from build123d import *

# Parameters (mm, degrees)
CUT_EXTRUDE1_REACH  = 155.838
SKETCH2_R           = 1.5
SKETCH3_R           = 110
SKETCH3_R_2         = 85
SKETCH3_R_3         = 2.5
BOSS_EXTRUDE1_DEPTH = 5


with BuildPart() as part:
    # Sketch1 → Revolve1 (revolve)
    with BuildSketch(Plane.XY, mode=Mode.PRIVATE) as revolve1_sk:
        Polygon((80, 0), (80, 88), (6, 88), (6, 96), (25, 96), (25, 93), (35, 93), (35, 100), (85, 100), (85, 0), align=None)
    revolve(revolve1_sk.sketch.rotate(Axis((0, 0, 0), (0, 1, 0)), 90), axis=Axis((0, 0, 0), (0, 1, 0)))

    # Sketch2 → Cut-Extrude1 (cut, up to next)
    with BuildSketch(Plane(origin=(0, 96, 0), x_dir=(1, 0, 0), z_dir=(0, 1, 0)), mode=Mode.PRIVATE) as cut_extrude1_sk1:
        with Locations(Location((0, 10.052527236, 0), (0, 0, 270))):
            Circle(SKETCH2_R)
    cut_extrude1_tool1 = extrude(cut_extrude1_sk1.sketch, amount=-CUT_EXTRUDE1_REACH, mode=Mode.PRIVATE) & part.part
    # Sketch2 → Cut-Extrude1 (cut, up to next)
    with BuildSketch(Plane(origin=(0, 96, 0), x_dir=(1, 0, 0), z_dir=(0, 1, 0)), mode=Mode.PRIVATE) as cut_extrude1_sk2:
        with Locations(Location((-9.888059839, -1.883815278, 0), (0, 0, 270))):
            Circle(SKETCH2_R)
    cut_extrude1_tool2 = extrude(cut_extrude1_sk2.sketch, amount=-CUT_EXTRUDE1_REACH, mode=Mode.PRIVATE) & part.part
    # Sketch2 → Cut-Extrude1 (cut, up to next)
    with BuildSketch(Plane(origin=(0, 96, 0), x_dir=(1, 0, 0), z_dir=(0, 1, 0)), mode=Mode.PRIVATE) as cut_extrude1_sk3:
        with Locations(Location((-4.4752587, -16.407987676, 0), (0, 0, 270))):
            Circle(SKETCH2_R)
    cut_extrude1_tool3 = extrude(cut_extrude1_sk3.sketch, amount=-CUT_EXTRUDE1_REACH, mode=Mode.PRIVATE) & part.part
    # Sketch2 → Cut-Extrude1 (cut, up to next)
    with BuildSketch(Plane(origin=(0, 96, 0), x_dir=(1, 0, 0), z_dir=(0, 1, 0)), mode=Mode.PRIVATE) as cut_extrude1_sk4:
        with Locations(Location((15.268544691, 7.491431306, 0), (0, 0, 270))):
            Circle(SKETCH2_R)
    cut_extrude1_tool4 = extrude(cut_extrude1_sk4.sketch, amount=-CUT_EXTRUDE1_REACH, mode=Mode.PRIVATE) & part.part
    add(cut_extrude1_tool1.solids().sort_by_distance((0, 96, -10.052527))[0], mode=Mode.SUBTRACT)
    add(cut_extrude1_tool2.solids().sort_by_distance((-9.88806, 96, 1.883815))[0], mode=Mode.SUBTRACT)
    add(cut_extrude1_tool3.solids().sort_by_distance((-4.475259, 96, 16.407988))[0], mode=Mode.SUBTRACT)
    add(cut_extrude1_tool4.solids().sort_by_distance((15.268545, 96, -7.491431))[0], mode=Mode.SUBTRACT)

    # Sketch3 → Boss-Extrude1 (add)
    with BuildSketch(Plane.XZ):
        with Locations(Location((0, 0, 0), (0, 0, 270))):
            Circle(SKETCH3_R)
        with Locations(Location((0, 0, 0), (0, 0, 270))):
            Circle(SKETCH3_R_2, mode=Mode.SUBTRACT)
        with Locations(Location((0, 97.5, 0), (0, 0, 270))):
            Circle(SKETCH3_R_3, mode=Mode.SUBTRACT)
        with Locations(Location((97.5, 0, 0), (0, 0, 270))):
            Circle(SKETCH3_R_3, mode=Mode.SUBTRACT)
        with Locations(Location((0, -97.5, 0), (0, 0, 270))):
            Circle(SKETCH3_R_3, mode=Mode.SUBTRACT)
        with Locations(Location((-97.5, 0, 0), (0, 0, 270))):
            Circle(SKETCH3_R_3, mode=Mode.SUBTRACT)
    extrude(amount=-BOSS_EXTRUDE1_DEPTH)


solid = part.part
Source: CAD feature listing. Evaluate the final solid. Frame: model axes, mm. A direction names the side the tool comes from. Coordinates: 2 decimals unless noted, no trailing zeros. Loops run counter-clockwise (first coordinate to the right, second up) from the corner with the lowest first, then second, coordinate; pieces in that order, holes last. Notation, with made-up numbers: (62.5, -8) -> (94.5, -8) arc R24 ccw to (94.5, 8) -> close; hole circle Ø6 at (54.25, 50). An arc over 180 degrees is marked (long way). Answer in a Markdown table with one row per item. Add a question column.
Q1. Pull-direction query (X, two-part tool) for faces 4 (the face through (25, 5, 82)), 5 (the face through (100, 2, 0)), 6 (the face through (-97.59, 2.46, -50.76)); classes: pulls with the +X half, pulls with the -X half, needs draft (parallel to the pull), parting line crosses it, or undercut.
Q2. Section B-B on z = -70.5. Return the cut outline in (x, y).
Q3. Contact query for flat-ended pins moving along their axis: pin 1 Ø2 at (y, z) = (14, 45.5) entering from -X; pin 2 Ø3 at (x, y) = (-32, 47) entering from -Z; pin 3 Ø3 at (x, z) = (97.5, 0) entering from -Y; pin 4 Ø10 at (x, y) = (19, 26) entering from +Z. Output: stop coordinate, or through.
Q4. Ray query, line 1 along X through (y, z) = (94, 0); line 2 along Y through (x, z) = (15, -85.5); line 3 along Y through (x, z) = (63.5, -5.5). Return the intervals inside material, ascending.
Q5. Section C-C on y = 19. Return the cut outline in (x, z), and give its area (3 significant figures).
Q6. Section A-A on x = 57.5. Return the cut outline in (y, z) (3 decimals), and give its area (3 significant figures).
Q7. Section D-D on z = 11.5. Return the cut outline in (x, y), and give its area (3 significant figures).
Q8. Reachability of faces 1 (the face through (-3.517, 44.616, 79.923)), 2 (the face through (37, 100, -1)), 3 (the face through (34.168, 96.549, 7.587)) from +Z, -Z, +X, -X, +Y, -Y: full face, straight path, thin tool, end or side. Return the list, or none.
Computed values:
| question | item | result |
|---|---|---|
| 1 | face 4 | needs draft |
| 1 | face 5 | undercut |
| 1 | face 6 | parting line crosses it |
| 2 | outline | (-84.44, 0) -> (-37.81, 0) -> (-37.81, 88) -> (37.81, 88) -> (37.81, 0) -> (84.44, 0) -> (84.44, 5) -> (47.48, 5) -> (47.48, 100) -> (-47.48, 100) -> (-47.48, 5) -> (-84.44, 5) -> close |
| 3 | pin 1 | stops at x = -72.42 |
| 3 | pin 2 | stops at z = -79.34 |
| 3 | pin 3 | passes through |
| 3 | pin 4 | stops at z = 83.84 |
| 4 | line 1 | x = -85 to -35, -25 to -6, 6 to 25, 35 to 85 |
| 4 | line 2 | y = 0 to 5 |
| 4 | line 3 | y = 88 to 100 |
| 5 | outline | circle Ø170 at (0, 0); hole circle Ø160 at (0, 0) |
| 5 | area | 2,590 mm^2 |
| 6 | outline | (0, -93.775) -> (5, -93.775) -> (5, -62.6) -> (100, -62.6) -> (100, 62.6) -> (5, 62.6) -> (5, 93.775) -> (0, 93.775) -> (0, 55.621) -> (88, 55.621) -> (88, -55.621) -> (0, -55.621) -> close |
| 6 | area | 3,040 mm^2 |
| 7 | outline | (-109.4, 0) -> (-79.17, 0) -> (-79.17, 88) -> (79.17, 88) -> (79.17, 0) -> (109.4, 0) -> (109.4, 5) -> (84.22, 5) -> (84.22, 100) -> (33.06, 100) -> (33.06, 93) -> (22.2, 93) -> (22.2, 96) -> (-22.2, 96) -> (-22.2, 93) -> (-33.06, 93) -> (-33.06, 100) -> (-84.22, 100) -> (-84.22, 5) -> (-109.4, 5) -> close |
| 7 | area | 2,830 mm^2 |
| 8 | face 1 | -Y |
| 8 | face 2 | +Z, -Z, +X, -X, +Y |
| 8 | face 3 | +Y |
